Geometry check sheet. Reference: drawing and pictorial views, mm from the part's lowest x, y, z. Round coordinates to 2 decimals unless told otherwise and drop trailing zeros. Order: outer loops, then holes, each group sorted by start corner. A loop starts at its lowest first (then second) coordinate and runs counter-clockwise, first axis right, second up.
(1) Release check for a two-part mould opening along X. For the marked faces 1 and 2 record: +X half, -X half, draft (parallel to the pull), parting line (faces both ways), or undercut.
(2) Sectioned sample at B-B (x = 605). Record the boundary of the cut face in (y, z), plus the area to 3 significant figures.
(3) Sectioned sample at A-A (y = 181). Record the boundary of the cut face in (x, z).
(4) Material ranges on line 1 along X through (y, z) = (262.5, 19); line 2 along X through (y, z) = (417, 30.5); line 3 along Z through (x, y) = (545, 400.5), recorded low to high.
(5) Go/stop test with flat-tipped pins: pin 1 (5 mm diameter, centred on x = 336.5, y = 375.5, fed in from -Z); pin 2 (20 mm diameter, centred on x = 253, z = 24.5, fed in from -Y); pin 3 (3 mm diameter, centred on x = 325, z = 37, fed in from +Y). Record where each tip stops, or that it passes through.
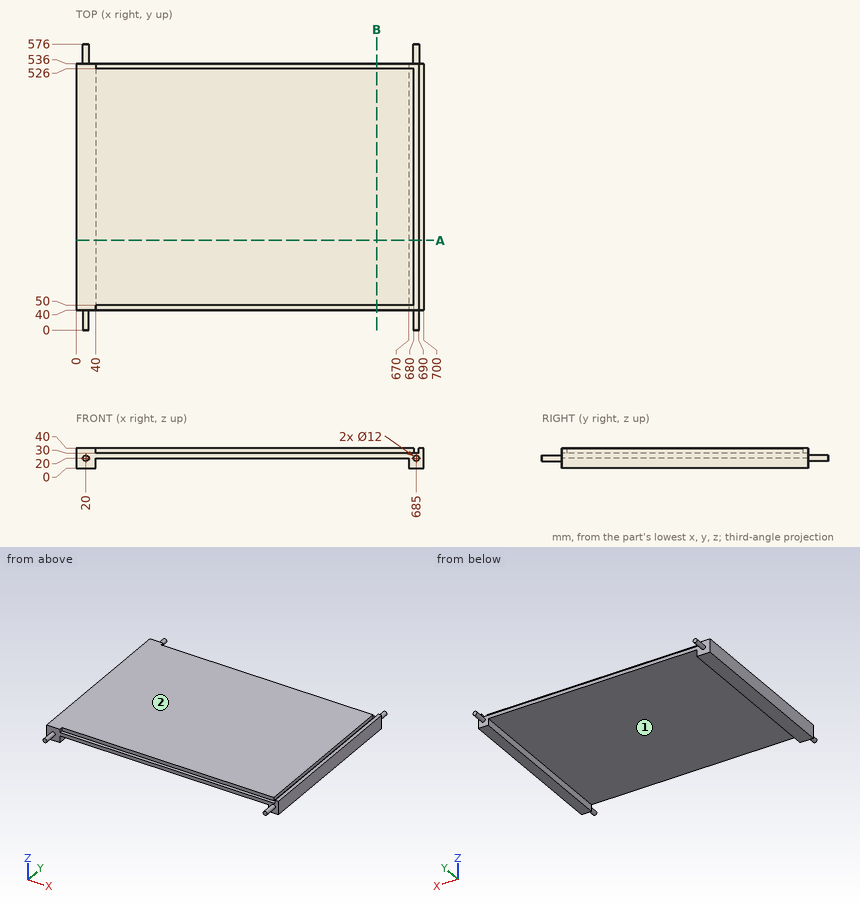
Answer below:
1. face 1: undercut
1. face 2: draft
2. outline: (40, 20) - (536, 20) - (536, 30) - (526, 30) - (526, 40) - (50, 40) - (50, 30) - (40, 30) - close
2. area: 9,720 mm2
3. outline: (0, 0) - (40, 0) - (40, 20) - (670, 20) - (670, 0) - (700, 0) - (700, 40) - (690, 40) - (690, 30) - (680, 30) - (680, 40) - (0, 40) - close
4. line 1: x = 0 to 40, 670 to 700
4. line 2: x = 0 to 680, 690 to 700
4. line 3: z = 20 to 40
5. pin 1: stops at z = 20
5. pin 2: stops at y = 40
5. pin 3: stops at y = 526
